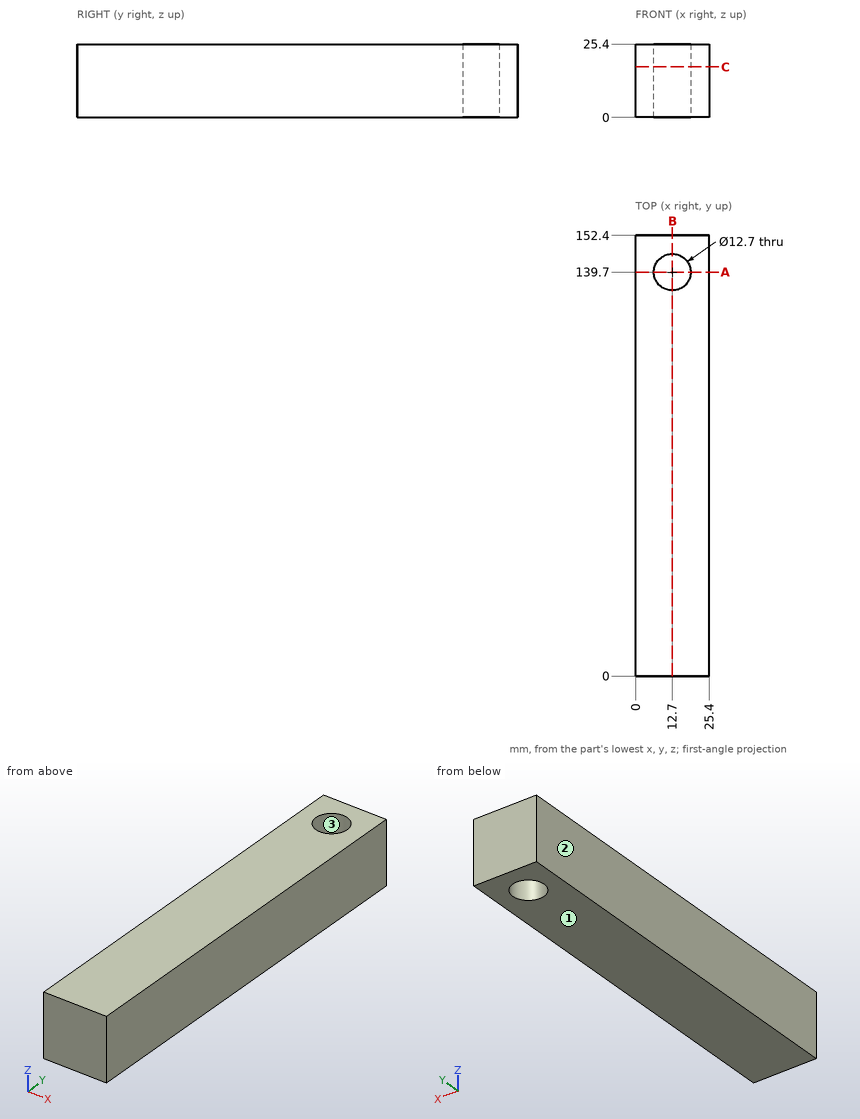
Can you work these out from the drawing? Everything is in mm from the part's minimum corner. Give positions to 0.01 mm unless a question says otherwise; leave off trailing zeros. Loops run counter-clockwise (first coordinate to the right, second up) from the corner with the lowest first, then second, coordinate; pieces in that order, holes last. Notation, with made-up numbers: M 18.5,35.25 L 60.5,35.25 A31 ccw 60.5,65.25 Z; hole C -16.5,-9 d1. An arc over 180 degrees is marked long. Use CSV: the item, a comma, the result in double quotes. Start each with the question number.
1. Imagine slicing it at B-B, the plane x = 12.7. Write out the boundary of the cut face in (y, z).
2. If I drill on L1, parallel to Y at x = 12.7, z = 8.25; L2, parallel to Y at x = 7.5, z = 1.5, over which ranges is the centre line in solid material (lowest first)?
3. If we mould it in two halves opening along X, with no side actions, what happens to the marked faces 1, 2 and 3? For each: released by +X, released by -X, zero draft, split by the parting line, or undercut.
4. Imagine slicing it at C-C, the plane z = 17.5. Write out the boundary of the cut face in (x, y), plus the area to 3 significant figures.
5. Imagine slicing it at A-A, the plane y = 139.7. Write out the boundary of the cut face in (x, z).
6. For P1, Ø6, axis at x = 3, z = 8.5, coming from the -Y side, with a flat end and sliding along its axis, tell me the tip position at first contact or that it passes through.
Response values:
1,outline,"M 0,0 L 133.35,0 L 133.35,25.4 L 0,25.4 Z; M 146.05,0 L 152.4,0 L 152.4,25.4 L 146.05,25.4 Z"
2,L1,"0 to 133.35, 146.05 to 152.4"
2,L2,"0 to 136.06, 143.34 to 152.4"
3,face 1,"zero draft"
3,face 2,"released by -X"
3,face 3,"undercut"
4,outline,"M 0,0 L 25.4,0 L 25.4,152.4 L 0,152.4 Z; hole C 12.7,139.7 d12.7"
4,area,"3,740 mm^2"
5,outline,"M 0,0 L 6.35,0 L 6.35,25.4 L 0,25.4 Z; M 19.05,0 L 25.4,0 L 25.4,25.4 L 19.05,25.4 Z"
6,P1,"y = 0"
